Study the drawing (mm; zero at the part's minimum x, y, z) and answer. A direction names the side the tool comes from. Give positions to 0.01 mm unless a question says otherwise; leave off trailing zeros. Write each loop counter-clockwise with the first axis right and the second up, starting at its lowest first coordinate (ties: lowest second). Pieces come first, ordered by that corner, then holes. Notation, with made-up numbers: (86, 3.5) - (140, 3.5) arc R24 ccw to (140, 35.5) - close; hole circle Ø2 at (49.25, 15.5). An arc over 180 degrees is marked (long way). Answer as CSV lines item,"result".
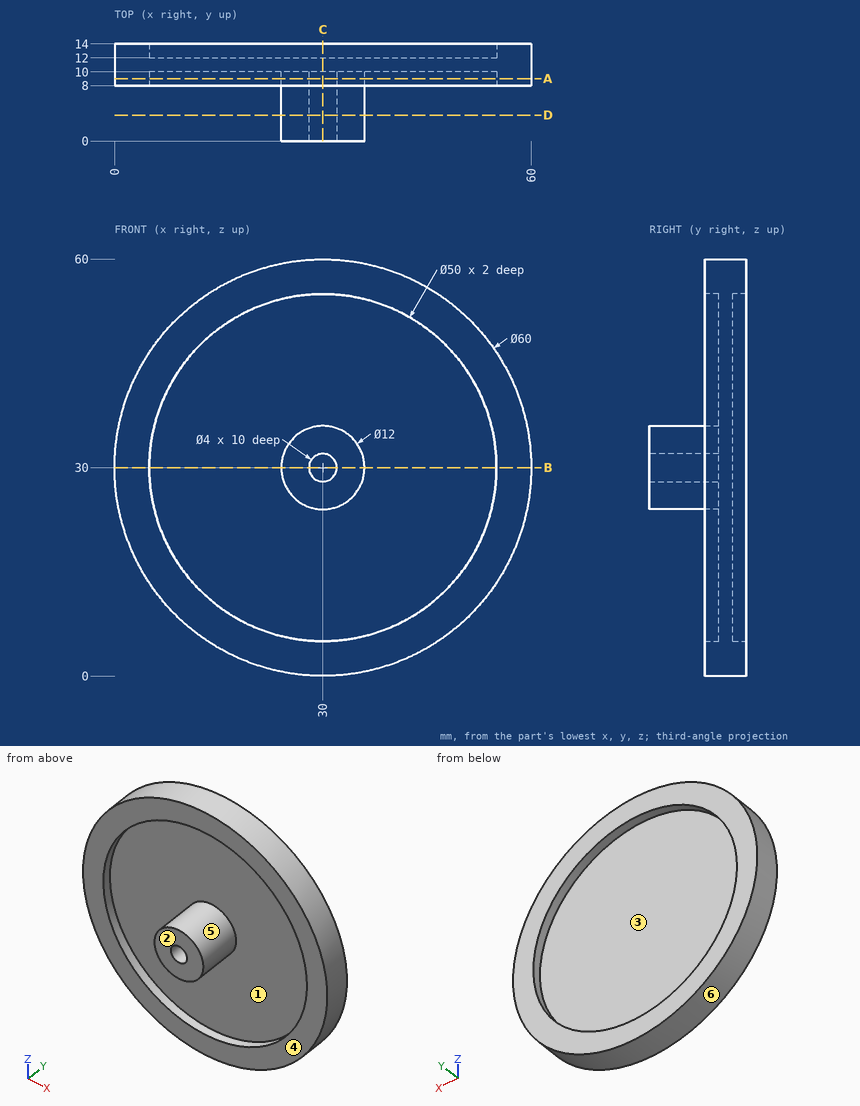
(1) Find the intervals of material crossed by L1, parallel to X at y = 8.25, z = 30; L2, parallel to Z at x = 25.5, y = 9.5; L3, parallel to X at y = 13.45, z = 30, in increasing order.
Worked out:
L1,"x = 0 to 5, 24 to 28, 32 to 36, 55 to 60"
L2,"z = 0.34 to 5.41, 26.03 to 33.97, 54.59 to 59.66"
L3,"x = 0 to 5, 55 to 60"
(2) A cutting plane is placed at D-D (y = 3.75). Write down the section's boundary in (x, z), and give its area (3 significant figures).
Worked out:
outline,"circle Ø12 at (30, 30); hole circle Ø4 at (30, 30)"
area,"101 mm^2"
(3) A cutting plane is placed at B-B (z = 30). Write down the section's boundary in (x, y).
Worked out:
outline,"(0, 8) - (5, 8) - (5, 10) - (24, 10) - (24, 0) - (28, 0) - (28, 10) - (32, 10) - (32, 0) - (36, 0) - (36, 10) - (55, 10) - (55, 8) - (60, 8) - (60, 14) - (55, 14) - (55, 12) - (5, 12) - (5, 14) - (0, 14) - close"
(4) For the marked faces 1, 2 and 3, determine the directions among +Z, -Z, +X, -X, +Y, -Y from which every point of the face is accessible in a straight line to the end or side of a thin tool.
Worked out:
face 1,"-Y"
face 2,"+Z, -Z, +X, -X, -Y"
face 3,"+Y"
(5) A cutting plane is placed at A-A (y = 9). Write down the section's boundary in (x, z), and give its area (3 significant figures).
Worked out:
outline,"circle Ø60 at (30, 30); circle Ø12 at (30, 30); hole circle Ø50 at (30, 30); hole circle Ø4 at (30, 30)"
area,"964 mm^2"
(6) The mould has two halves that part along Z. Classify the marked faces 4, 5 and 6: +Z half, -Z half, draft (parallel to the pull), parting line (faces both ways), or undercut.
Worked out:
face 4,"draft"
face 5,"undercut"
face 6,"parting line"
(7) Each of these flat-tipped pins is pushed along its axis until it touches: P1, Ø2, axis at x = 37.5, z = 26.5, coming from the -Y side; P2, Ø2, axis at x = 48.5, z = 26, coming from the +Y side; P3, Ø4, axis at x = 37, y = 1.5, coming from the +Z side. Where does it stop, or does it pass through?
Worked out:
P1,"stops at y = 10"
P2,"stops at y = 12"
P3,"stops at z = 33.32"
(8) A cutting plane is placed at C-C (x = 30). Write down the section's boundary in (y, z), and give its area (3 significant figures).
Worked out:
outline,"(0, 24) - (10, 24) - (10, 5) - (8, 5) - (8, 0) - (14, 0) - (14, 5) - (12, 5) - (12, 55) - (14, 55) - (14, 60) - (8, 60) - (8, 55) - (10, 55) - (10, 36) - (0, 36) - (0, 32) - (10, 32) - (10, 28) - (0, 28) - close"
area,"240 mm^2"
